Read the model definition and answer for the solid it produces. Units are mm, in the model's axes. A direction names the side the tool comes from. Coordinates: 2 decimals unless noted, no trailing zeros. Write each loop counter-clockwise with the first axis right and the second up, starting at its lowest first coordinate (ties: lowest second). Pieces come first, ordered by that corner, then holes. Notation, with made-up numbers: (52.5, -10) -> (70.5, -10) arc R16 ccw to (70.5, -1) -> close; hole circle Ø11 at (-14.5, -11). An arc over 180 degrees is marked (long way). Answer as a JSON object with one key per item and string values. Group by question number.
(1) Find section A-A (z = 6). Give the vertices of the cut face in (x, y) (3 decimals).
(2) Find section D-D (x = 0). Give the vertices of the cut face in (y, z) (3 decimals), then the cut area to 3 significant figures.
(3) Find section C-C (y = 0.9). Count the separate pieces of the cut face and the enclosed holes in it, then the cut area to 3 significant figures.
(4) Which of the six approach directions +Z, -Z, +X, -X, +Y, -Y give full straight-line access (tool end or side, diameter ignored) to faces 1 (the face through (-16, 1, 13.15)), 2 (the face through (-13.26, 1.01, 0.05)), 3 (the face through (21.6, 0.74, 16.64))?
(5) Find section B-B (x = 13). Give the vertices of the cut face in (y, z).
(6) For a pull along X with two mould halves and no side action, classify faces 4 (the face through (8.374, 1.007, -0.091)), 5 (the face through (22.5, 1, 0)), 6 (the face through (0, 0, -4)), 7 (the face through (-16, 1, 10.85)) as +X half, -X half, draft (parallel to the pull), parting line (faces both ways), or undercut.
(7) Straight lines are drawn through the part: L1, parallel to Z at x = -14.5, y = 0.9; L2, parallel to X at y = 1, z = 6 (3 decimals); L3, parallel to Z at x = -17.5, y = 1.1. For each, find the intervals that lie inside material, in ascending order.
(8) Flat-ended cylindrical pins translate along their axes: P1, Ø0.8, axis at x = -16.5, y = 0.5, coming from the +Z side; P2, Ø3, axis at x = 19.5, z = 0, coming from the +Y side; P3, Ø2.5, axis at x = 4.5, z = 0, coming from the +Y side; P4, Ø1.1, axis at x = -2.5, z = 0, coming from the -Y side. Find the tip coordinate at first contact, or state that the pin passes through.
from build123d import *

# Parameters (mm, degrees)
SALIENTE_EXTRUIR1_DEPTH = 1.5
CORTAR_EXTRUIR1_DEPTH   = 1
CROQUIS3_R              = 1.125
CROQUIS3_W              = 3.8
CROQUIS3_H              = 2.3
CORTAR_EXTRUIR2_DEPTH   = 1
CROQUIS4_R              = 0.875
CORTAR_EXTRUIR3_DEPTH   = 10


with BuildPart() as part:
    # Croquis1 → Saliente-Extruir1 (new body)
    with BuildSketch(Plane(origin=(0, 0, 0), x_dir=(1, 0, 0), z_dir=(0, 1, 0))):
        with BuildLine():
            Line((-14.5, -17.5), (19.5, -17.5))
            ThreePointArc((19.5, -17.5), (21.621320344, -16.621320344), (22.5, -14.5))
            Line((22.5, -14.5), (22.5, 14.5))
            ThreePointArc((22.5, 14.5), (21.621320344, 16.621320344), (19.5, 17.5))
            Line((19.5, 17.5), (-14.5, 17.5))
            ThreePointArc((-14.5, 17.5), (-20.156854249, 15.156854249), (-22.5, 9.5))
            Line((-22.5, 9.5), (-22.5, -9.5))
            ThreePointArc((-22.5, -9.5), (-20.156854249, -15.156854249), (-14.5, -17.5))
        make_face()
    extrude(amount=SALIENTE_EXTRUIR1_DEPTH)

    # Croquis2 → Cortar-Extruir1 (cut)
    with BuildSketch(Plane(origin=(0, 1.5, 0), x_dir=(1, 0, 0), z_dir=(0, 1, 0))):
        with BuildLine():
            Line((-11.235477419, 2.247698909), (4.09625, 3.853908527))
            ThreePointArc((4.09625, 3.853908527), (8.375, 0), (4.09625, -3.853908527))
            Line((4.09625, -3.853908527), (-11.235477419, -2.247698909))
            ThreePointArc((-11.235477419, -2.247698909), (-13.26, 0), (-11.235477419, 2.247698909))
        make_face()
    extrude(amount=-CORTAR_EXTRUIR1_DEPTH, mode=Mode.SUBTRACT)

    # Croquis3 → Cortar-Extruir2 (cut, symmetric)
    with BuildSketch(Plane(origin=(0, 0.5, 0), x_dir=(1, 0, 0), z_dir=(0, 1, 0))):
        with Locations(Location((4.5, 0, 0), (0, 0, 270))):
            Circle(CROQUIS3_R)
        with Locations(Location((19.5, 6, 0), (0, 0, 270))):
            Circle(CROQUIS3_R)
        with Locations(Location((19.5, -6, 0), (0, 0, 270))):
            Circle(CROQUIS3_R)
        with Locations(Location((19.5, 0, 0), (0, 0, 270))):
            Circle(CROQUIS3_R)
        with Locations((-15.697233885, 8.65)):
            Rectangle(CROQUIS3_W, CROQUIS3_H)
        with Locations((-15.697233885, -12)):
            Rectangle(CROQUIS3_W, CROQUIS3_H)
        with Locations((12.302766115, -12)):
            Rectangle(CROQUIS3_W, CROQUIS3_H)
        with Locations((12.302766115, 8.65)):
            Rectangle(CROQUIS3_W, CROQUIS3_H)
    extrude(amount=CORTAR_EXTRUIR2_DEPTH, both=True, mode=Mode.SUBTRACT)

    # Croquis4 → Cortar-Extruir3 (cut)
    with BuildSketch(Plane(origin=(0, 1.5, 0), x_dir=(1, 0, 0), z_dir=(0, 1, 0))):
        with Locations(Location((0, 0, 0), (0, 0, 270))):
            Circle(CROQUIS4_R)
        with Locations(Location((-5, 0, 0), (0, 0, 270))):
            Circle(CROQUIS4_R)
        with Locations(Location((-2.5, 0, 0), (0, 0, 270))):
            Circle(CROQUIS4_R)
        with Locations(Location((-7.5, 0, 0), (0, 0, 270))):
            Circle(CROQUIS4_R)
        with Locations(Location((-10, 0, 0), (0, 0, 270))):
            Circle(CROQUIS4_R)
    extrude(amount=-CORTAR_EXTRUIR3_DEPTH, mode=Mode.SUBTRACT)


solid = part.part
Results below:
{
 "1": {"outline": "(-22.5, 0) -> (18.375, 0) -> (18.375, 1.5) -> (-22.5, 1.5) -> close; (20.625, 0) -> (22.5, 0) -> (22.5, 1.5) -> (20.625, 1.5) -> close"},
 "2": {"outline": "(0, -17.5) -> (1.5, -17.5) -> (1.5, -3.425) -> (0.5, -3.425) -> (0.5, -0.875) -> (0, -0.875) -> close; (0, 0.875) -> (0.5, 0.875) -> (0.5, 3.425) -> (1.5, 3.425) -> (1.5, 17.5) -> (0, 17.5) -> close", "area": "44.8 mm2"},
 "3": {"separate pieces": "1", "enclosed holes": "8", "area": "1,370 mm2"},
 "4": {"face 1": "+Y, -Y", "face 2": "+Y", "face 3": "+Z, +X, +Y, -Y"},
 "5": {"outline": "(0, -17.5) -> (1.5, -17.5) -> (1.5, -9.8) -> (0, -9.8) -> close; (0, -7.5) -> (1.5, -7.5) -> (1.5, 10.85) -> (0, 10.85) -> close; (0, 13.15) -> (1.5, 13.15) -> (1.5, 17.5) -> (0, 17.5) -> close"},
 "6": {"face 4": "undercut", "face 5": "+X half", "face 6": "draft", "face 7": "undercut"},
 "7": {"L1": "z = -17.5 to -9.8, -7.5 to 10.85, 13.15 to 17.5", "L2": "x = -22.5 to 18.375, 20.625 to 22.5", "L3": "z = -16.92 to -9.8, -7.5 to 10.85, 13.15 to 16.92"},
 "8": {"P1": "stops at z = 17.34", "P2": "stops at y = 1.5", "P3": "stops at y = 0.5", "P4": "passes through"}
}
